Design review of the part built by this model. Coordinates are the model's own, in mm. A direction names the side the tool comes from. Give positions to 0.01 mm unless a question says otherwise; leave off trailing zeros. Loops run counter-clockwise (first coordinate to the right, second up) from the corner with the lowest first, then second, coordinate; pieces in that order, holes last. Notation, with made-up numbers: M 69,16.5 L 85,16.5 A10 ccw 85,32.5 Z; hole C -38,-3 d3. An arc over 180 degrees is marked long. Use CSV: the item, a comma, the result in double quotes.
from build123d import *

# Parameters (mm, degrees)
F0_W     = 12.5
F0_H     = 4.5
F1_DEPTH = 0.5
F2_W     = 12.5
F2_H     = 2
F3_DEPTH = 8.5
F5_DEPTH = 12.5


with BuildPart() as f1:
    # F0 (on Top) → F1 (new body)
    with BuildSketch(Plane.XY):
        Rectangle(F0_W, F0_H)
    extrude(amount=F1_DEPTH)

    # F2 (on face) → F3 (join)
    with BuildSketch(Plane.XY.offset(0.5)):
        with Locations((0, 1.25)):
            Rectangle(F2_W, F2_H)
    extrude(amount=F3_DEPTH)

    # F4 (on face) → F5 (join)
    with BuildSketch(Plane(origin=(-6.25, 0, 0), x_dir=(0, -1, 0), z_dir=(-1, 0, 0))):
        with BuildLine():
            ThreePointArc((3.70586, -10.21875), (5.396071, -8.123437), (6, -5.5))
            ThreePointArc((6, -5.5), (4.974937, -2.145898), (2.25, 0.062149))
            Line((2.25, 0.062149), (2.25, 0))
            Line((2.25, 0), (-2.25, 0))
            Line((-2.25, 0), (-2.25, 0.062149))
            ThreePointArc((-2.25, 0.062149), (-5.940731, -4.658743), (-3.70586, -10.21875))
            ThreePointArc((-3.70586, -10.21875), (-2.013298, -1.651378), (5.25, -6.5))
            ThreePointArc((5.25, -6.5), (4.848622, -8.513298), (3.70586, -10.21875))
        make_face()
    extrude(amount=-F5_DEPTH)


solid = f1.part
(1) Clearance check with flat-ended pins moving along their axes: P1, Ø3, axis at y = -1, z = -8, coming from the +X side (1 decimal); P2, Ø0.8, axis at x = 1, y = -0.5, coming from the +Z side; P3, Ø6, axis at x = 1.5, y = 3, coming from the -Z side; P4, Ø3, axis at x = -2, z = 1, coming from the -Y side. State where each tip first meets the part, or that it passes through.
A:
P1,"through"
P2,"z = 0.5"
P3,"z = -10.22"
P4,"y = -3.32"
(2) Machinability: for faces 1 (the flat face through (0, 0.25, 5)), 2 (the cylindrical face through (-0.088, 5.928, -4.572)), 3 (the flat face through (0, 2.25, 4)), which of the approach directions +Z, -Z, +X, -X, +Y, -Y give a long, thin tool a straight path to every point of the face, cutting with its end or side? Answer none if there is none.
A:
face 1,"+Z, +X, -X, -Y"
face 2,"+X, -X, +Y"
face 3,"+Z, +X, -X, +Y"
(3) We need section D-D on y = 0. State the section outline as (x, z) points, then the cut area to 3 significant figures.
A:
outline,"M -6.25,-1.25 L 6.25,-1.25 L 6.25,0.5 L -6.25,0.5 Z"
area,"21.9 mm²"
(4) We need section B-B on z = -7.75. State the section outline as (x, y) points, then the cut area to 3 significant figures.
A:
outline,"M -6.25,-5.56 L 6.25,-5.56 L 6.25,-5.1 L -6.25,-5.1 Z; M -6.25,5.1 L 6.25,5.1 L 6.25,5.56 L -6.25,5.56 Z"
area,"11.6 mm²"
(5) We need section C-C on x = 5.25. State the section outline as (y, z) points.
A:
outline,"M -6,-5.5 A6 ccw -3.71,-10.22 A5.25 cw -5.25,-6.5 A5.25 cw long 3.71,-10.22 A6 ccw 2.25,0.06 L 2.25,9 L 0.25,9 L 0.25,0.5 L -2.25,0.5 L -2.25,0.06 A6 ccw Z"
(6) Wall thickness on line 1 along Z through (x, y) = (0.75, 0); line 2 along Y through (x, z) = (4, 7.5); line 3 along Y through (x, z) = (4, -3.5): over which ranges is each line inside the solid? List them lowest first. Write a range as [from, to].
A:
line 1,"[-1.25, 0.5]"
line 2,"[0.25, 2.25]"
line 3,"[-5.66, -4.31], [4.31, 5.66]"
(7) We need section A-A on y = -4.5. State the section outline as (x, z) points, then the cut area to 3 significant figures.
A:
outline,"M -6.25,-9.47 L 6.25,-9.47 L 6.25,-9.2 L -6.25,-9.2 Z; M -6.25,-3.8 L 6.25,-3.8 L 6.25,-1.53 L -6.25,-1.53 Z"
area,"31.6 mm²"
